from build123d import *

# Parameters (mm, degrees)
EXTRUDE_START          = 0.1
EXTRUDE_1_DEPTH        = 70.5
SKETCH_3_W             = 0.4
SKETCH_3_H             = 10
CUT_EXTRUDE_1_DEPTH    = 89.958131389
EXTRUDE_START_2        = 0.3
EXTRUDE_2_DEPTH        = 6.4
EXTRUDE_3_REACH        = 103.657
EXTRUDE_3_START_RADIUS = 28
EXTRUDE_3_END_RADIUS   = 28
SKETCH_5_W             = 8.845499788
SKETCH_5_H             = 0.6
SKETCH_6_W             = 1.2
SKETCH_6_H             = 70.5
EXTRUDE_4_DEPTH        = 2
SKETCH_7_W             = 7.03
SKETCH_7_H             = 10.06
CUT_EXTRUDE_2_DEPTH    = 2


# Read off the part's stored shape, not the designer's step: Бобышка-Вытянуть2
with BuildPart() as part:
    # Эскиз1 → Бобышка-Вытянуть1 (new body)
    with BuildSketch(Plane.XY.offset(EXTRUDE_START)):
        with BuildLine():
            Line((20.652219826, -28.8), (-17.823198335, -28.8))
            ThreePointArc((-17.823198335, -28.8), (-37.586801245, -20.634313701), (-45.823019763, -0.9))
            Line((-45.823019763, -0.9), (-41.823019763, -0.9))
            Line((-41.823019763, -0.9), (-41.823019763, -2.1))
            Line((-41.823019763, -2.1), (-44.591649915, -2.1))
            ThreePointArc((-44.591649915, -2.1), (-36.308327493, -20.204638621), (-17.823198335, -27.6))
            Line((-17.823198335, -27.6), (19.452219826, -27.6))
            Line((19.452219826, -27.6), (19.452219826, -24.8))
            Line((19.452219826, -24.8), (20.652219826, -24.8))
            Line((20.652219826, -24.8), (20.652219826, -28.8))
        make_face()
    extrude(amount=EXTRUDE_1_DEPTH)

    # Эскиз3 → Вырез-Вытянуть1 (cut, through all)
    with BuildSketch(Plane(origin=(0, 0, 0), x_dir=(0, 0, -1), z_dir=(1, 0, 0))):
        with Locations((-44.05, -5.8)):
            Rectangle(SKETCH_3_W, SKETCH_3_H)
        with Locations((-26.65, -5.9)):
            Rectangle(SKETCH_3_W, SKETCH_3_H)
    extrude(amount=-CUT_EXTRUDE_1_DEPTH, mode=Mode.SUBTRACT)

    # Бобышка-Вытянуть2 outline → Бобышка-Вытянуть2 (add)
    with BuildSketch(Plane.XY.offset(31.886146776).offset(EXTRUDE_START_2)):
        with BuildLine():
            Line((-41.823019763, -2.1), (-41.023198335, -2.1))
            Line((-41.023198335, -2.1), (-41.023198335, 5.941310574))
            Line((-41.023198335, 5.941310574), (-41.423198335, 5.941310574))
            Line((-41.423198335, 5.941310574), (-43.62142157, 4.2))
            Line((-43.62142157, 4.2), (-43.62142157, 3.8))
            ThreePointArc((-43.62142157, 3.8), (-43.504264282, 3.517157288), (-43.22142157, 3.4))
            Line((-43.22142157, 3.4), (-42.223198335, 3.4))
            Line((-42.223198335, 3.4), (-42.223198335, -0.9))
            Line((-42.223198335, -0.9), (-41.823019763, -0.9))
            Line((-41.823019763, -0.9), (-41.823019763, -2.1))
        make_face()
    extrude(amount=EXTRUDE_2_DEPTH)

    # Бобышка-Вытянуть3: from a cylinder face, 103.657 long prism both ways, kept between that surface and its translate by the depth
    extrude_3_start = Plane(origin=(-17.823198335, -0.8, 35.35), z_dir=(0, 0, -1)) * Cylinder(EXTRUDE_3_START_RADIUS, 264.314, mode=Mode.PRIVATE)
    extrude_3_end = Plane(origin=(-18.323198335, -0.8, 35.35), z_dir=(0, 0, -1)) * Cylinder(EXTRUDE_3_END_RADIUS, 264.314, mode=Mode.PRIVATE)
    # Эскиз5 → Бобышка-Вытянуть3 (add, from a surface)
    with BuildSketch(Plane.ZY.offset(45.823198335), mode=Mode.PRIVATE) as extrude_3_sk1:
        with Locations((35.35, -3.019441342)):
            Rectangle(SKETCH_5_W, SKETCH_5_H)
    extrude_3_tool1 = extrude(extrude_3_sk1.sketch, amount=EXTRUDE_3_REACH, both=True, mode=Mode.PRIVATE)
    add(((extrude_3_tool1 - extrude_3_start) & extrude_3_end).solids().sort_by_distance((-45.34413, -3.019441, 35.35))[0])
    # Эскиз5 → Бобышка-Вытянуть3 (add, from a surface)
    with BuildSketch(Plane.ZY.offset(45.823198335), mode=Mode.PRIVATE) as extrude_3_sk2:
        with Locations((35.35, -4.419441342)):
            Rectangle(SKETCH_5_W, SKETCH_5_H)
    extrude_3_tool2 = extrude(extrude_3_sk2.sketch, amount=EXTRUDE_3_REACH, both=True, mode=Mode.PRIVATE)
    add(((extrude_3_tool2 - extrude_3_start) & extrude_3_end).solids().sort_by_distance((-45.34413, -3.019441, 35.35))[0])
    # Эскиз5 → Бобышка-Вытянуть3 (add, from a surface)
    with BuildSketch(Plane.ZY.offset(45.823198335), mode=Mode.PRIVATE) as extrude_3_sk3:
        with Locations((35.35, -5.819441342)):
            Rectangle(SKETCH_5_W, SKETCH_5_H)
    extrude_3_tool3 = extrude(extrude_3_sk3.sketch, amount=EXTRUDE_3_REACH, both=True, mode=Mode.PRIVATE)
    add(((extrude_3_tool3 - extrude_3_start) & extrude_3_end).solids().sort_by_distance((-45.34413, -3.019441, 35.35))[0])
    # Эскиз5 → Бобышка-Вытянуть3 (add, from a surface)
    with BuildSketch(Plane.ZY.offset(45.823198335), mode=Mode.PRIVATE) as extrude_3_sk4:
        Polygon((30.927250106, -7.519441342), (35.35, -9.519441342), (39.772749894, -7.519441342), (39.772749894, -6.919441342), (30.927250106, -6.919441342), align=None)
    extrude_3_tool4 = extrude(extrude_3_sk4.sketch, amount=EXTRUDE_3_REACH, both=True, mode=Mode.PRIVATE)
    add(((extrude_3_tool4 - extrude_3_start) & extrude_3_end).solids().sort_by_distance((-45.34413, -3.019441, 35.35))[0])

    # Эскиз6 → Бобышка-Вытянуть4 (add)
    with BuildSketch(Plane(origin=(0, -27.6, 0), x_dir=(1, 0, 0), z_dir=(0, 1, 0))):
        with Locations((-19.018158387, -35.35)):
            Rectangle(SKETCH_6_W, SKETCH_6_H)
        with Locations((17.134396076, -35.35)):
            Rectangle(SKETCH_6_W, SKETCH_6_H)
        Polygon((0.234396076, -8.7), (12.380116687, -8.7), (12.380116687, -2.5), (16.280116687, -2.5), (16.280116687, -0.1), (15.080116687, -0.1), (15.080116687, -1.3), (11.180116687, -1.3), (11.180116687, -7.5), (-4.619883313, -7.5), (-4.619883313, -1.3), (-8.519883313, -1.3), (-8.519883313, -0.1), (-9.719883313, -0.1), (-9.719883313, -2.5), (-5.819883313, -2.5), (-5.819883313, -8.7), (-1.118158387, -8.7), (-1.118158387, -70.6), (0.234396076, -70.6), align=None)
    extrude(amount=EXTRUDE_4_DEPTH)

    # Эскиз7 → Вырез-Вытянуть2 (cut)
    with BuildSketch(Plane(origin=(0, -0.9, 0), x_dir=(1, 0, 0), z_dir=(0, 1, 0))):
        with Locations((-40.908198335, -57.75)):
            Rectangle(SKETCH_7_W, SKETCH_7_H)
    extrude(amount=-CUT_EXTRUDE_2_DEPTH, mode=Mode.SUBTRACT)


solid = part.part
For this review, take the finished solid that the model builds, in its own axes (mm). A direction names the side the tool comes from. Give positions to 0.01 mm unless a question says otherwise; leave off trailing zeros. Loops run counter-clockwise (first coordinate to the right, second up) from the corner with the lowest first, then second, coordinate; pieces in that order, holes last.
Item 1: Take a section at C-C, the plane y = 0.5. State the section outline as (x, z) points, and give its area (3 significant figures).
Item 2: Draft analysis for pull direction Z (two halves, no side actions). For faces 1 (the flat face through (-15, -28, 70.6)), 2 (the flat face through (-42.223, 1, 35)), 3 (the flat face through (-17, -28, 0.1)), 4 (the flat face through (-45, -5, 43.85)), state which applies: +Z half, -Z half, draft (parallel to the pull), parting line (faces both ways), or undercut.
Item 3: Take a section at B-B, the plane x = -2.5. State the section outline as (y, z) points, and give its area (3 significant figures).
Item 4: Take a section at D-D, the plane x = -34.5. State the section outline as (y, z) points, and give its area (3 significant figures).
Item 5: Tool access review of faces 5 (the flat face through (17.734, -27, 36)), 6 (the flat face through (-41.023, 2, 35)), 7 (the flat face through (-45, -8.5, 33.1)), 8 (the flat face through (11.18, -27, 4)), 9 (the flat face through (14, -27, 2.5)): name each direction out of +Z, -Z, +X, -X, +Y, -Y from which nothing blocks a thin tool from reaching the whole face with its end or side.
Item 6: For line 1 along Y through (x, z) = (-1, 31.5); line 2 along Y through (x, z) = (7, 18.5); line 3 along X through (y, z) = (-4, 61), list the stretches that pass through material, from the lowest coordinate up.
Item 7: Take a section at A-A, the plane z = 60. State the section outline as (x, y) points.
Item 8: Insertion check: pin 1 (4.5 mm diameter, centred on x = -45, z = 56, fed in from +Y); pin 2 (4 mm diameter, centred on x = 12.5, z = 34.5, fed in from +Y); pin 3 (1.4 mm diameter, centred on x = -42.5, z = 18.5, fed in from -Y); pin 4 (3 mm diameter, centred on y = 1.5, z = 42.5, fed in from +X). Each pin has a flat end and moves straight along its axis. Give the tip position at first contact, or say it passes through.
Calculated:
1. outline: (-42.22, 32.19) - (-41.02, 32.19) - (-41.02, 38.59) - (-42.22, 38.59) - close
1. area: 7.68 mm2
2. face 1: +Z half
2. face 2: draft
2. face 3: -Z half
2. face 4: undercut
3. outline: (-28.8, 0.1) - (-27.6, 0.1) - (-27.6, 7.5) - (-25.6, 7.5) - (-25.6, 8.7) - (-27.6, 8.7) - (-27.6, 70.6) - (-28.8, 70.6) - close
3. area: 87.0 mm2
4. outline: (-23.29, 0.1) - (-21.78, 0.1) - (-21.78, 70.6) - (-23.29, 70.6) - close
4. area: 107 mm2
5. face 5: +Z, -Z, +Y
5. face 6: +Z, -Z, +X, +Y
5. face 7: -Z, -X, -Y
5. face 8: -Z, +Y
5. face 9: +Z, +Y
6. line 1: y = -28.8 to -25.6
6. line 2: y = -28.8 to -27.6
6. line 3: x = -45.64 to -44.43
7. outline: (-45.82, -0.9) arc R28 ccw to (-17.82, -28.8) - (20.65, -28.8) - (20.65, -24.8) - (19.45, -24.8) - (19.45, -27.6) - (17.73, -27.6) - (17.73, -25.6) - (16.53, -25.6) - (16.53, -27.6) - (0.23, -27.6) - (0.23, -25.6) - (-1.12, -25.6) - (-1.12, -27.6) - (-17.82, -27.6) arc R26.8 cw to (-18.42, -27.59) - (-18.42, -25.6) - (-19.62, -25.6) - (-19.62, -27.54) arc R26.8 cw to (-44.59, -2.1) - (-44.42, -2.1) - (-44.42, -0.9) - close
8. pin 1: stops at y = -0.9
8. pin 2: stops at y = -27.6
8. pin 3: stops at y = -15.26
8. pin 4: passes through
